The listing builds one solid part. Answer for the finished solid, in the listing's coordinates (mm). Face numbers are marked on the shaded views. A direction names the side the tool comes from. Coordinates: 2 decimals unless noted, no trailing zeros. Order: outer loops, then holes, each group sorted by start corner. A loop starts at its lowest first (then second) coordinate and runs counter-clockwise, first axis right, second up. Notation, with made-up numbers: (63.25, 71.5) -> (94.25, 71.5) arc R29 cw to (94.25, 110.5) -> close; hole circle Ø5 at (83, 7.5). An arc over 180 degrees is marked (long way). Return JSON: item names as keys, results as strings.
from build123d import *

# Parameters (mm, degrees)
SCHIZZO1_W                   = 20
SCHIZZO1_H                   = 15
SCHIZZO1_R                   = 1.75
ESTRUSIONE_ESTRUSIONE1_DEPTH = 5
SCHIZZO3_W                   = 20
SCHIZZO3_H                   = 5
ESTRUSIONE_ESTRUSIONE2_DEPTH = 13.5
SCHIZZO4_W                   = 20
SCHIZZO4_H                   = 5
ESTRUSIONE_ESTRUSIONE3_DEPTH = 17
RACCORDO1_R                  = 1


with BuildPart() as part:
    # Schizzo1 → Estrusione-Estrusione1 (new body)
    with BuildSketch(Plane.XY):
        Rectangle(SCHIZZO1_W, SCHIZZO1_H)
        with Locations((0, 2.5)):
            Circle(SCHIZZO1_R, mode=Mode.SUBTRACT)
    extrude(amount=ESTRUSIONE_ESTRUSIONE1_DEPTH)

    # Schizzo3 → Estrusione-Estrusione2 (add)
    with BuildSketch(Plane(origin=(0, 0, 0), x_dir=(-1, 0, 0), z_dir=(0, 0, -1))):
        with Locations((0, -5)):
            Rectangle(SCHIZZO3_W, SCHIZZO3_H)
    extrude(amount=ESTRUSIONE_ESTRUSIONE2_DEPTH)

    # Schizzo4 → Estrusione-Estrusione3 (add)
    with BuildSketch(Plane(origin=(0, -2.5, 0), x_dir=(1, 0, 0), z_dir=(0, 1, 0))):
        with Locations((0, 11)):
            Rectangle(SCHIZZO4_W, SCHIZZO4_H)
    extrude(amount=ESTRUSIONE_ESTRUSIONE3_DEPTH)

    # Raccordo1
    raccordo1_edges = [part.edges().sort_by_distance(p)[0] for p in [
        (0, -7.5, 5),
        (0, -7.5, -13.5),
        (0, 14.5, -13.5),
    ]]
    fillet(raccordo1_edges, radius=RACCORDO1_R)


solid = part.part
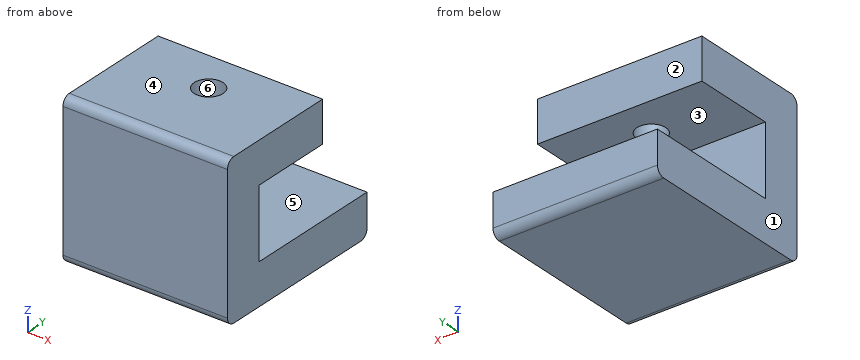
1. The part is cut by section A-A on y = 2.5. Give the vertices of the cut face in (x, z).
Answer block:
{"outline": "(-10, -13.5) -> (10, -13.5) -> (10, -8.5) -> (-10, -8.5) -> close; (-10, 0) -> (-1.75, 0) -> (-1.75, 5) -> (-10, 5) -> close; (1.75, 0) -> (10, 0) -> (10, 5) -> (1.75, 5) -> close"}
2. Determine the mould class of the marked faces 4, 5 and 6 for opening direction Z: pulls with the +Z half, pulls with the -Z half, needs draft (parallel to the pull), parting line crosses it, or undercut.
Answer block:
{"face 4": "pulls with the +Z half", "face 5": "undercut", "face 6": "needs draft"}
3. For the marked faces 1, 2 and 3, determine the directions among +Z, -Z, +X, -X, +Y, -Y from which every point of the face is accessible in a straight line to the end or side of a thin tool.
Answer block:
{"face 1": "+Z, -Z, -X, +Y, -Y", "face 2": "+Z, +X, -X, +Y", "face 3": "+X, -X, +Y"}
4. Each of these flat-tipped pins is pushed along its axis until it touches: pin 1 Ø4 at (y, z) = (10, 1.5) entering from +X; pin 2 Ø2.5 at (x, z) = (1.5, 3.5) entering from +Y; pin 3 Ø4 at (x, z) = (2, -6) entering from +Y. Where does it stop, or does it pass through?
Answer block:
{"pin 1": "passes through", "pin 2": "stops at y = 7.5", "pin 3": "stops at y = -2.5"}
5. The part is cut by section B-B on x = 0. Give the vertices of the cut face in (y, z), and give its area (3 significant figures).
Answer block:
{"outline": "(-7.5, -12.5) arc R1 ccw to (-6.5, -13.5) -> (13.5, -13.5) arc R1 ccw to (14.5, -12.5) -> (14.5, -8.5) -> (-2.5, -8.5) -> (-2.5, 0) -> (0.75, 0) -> (0.75, 5) -> (-6.5, 5) arc R1 ccw to (-7.5, 4) -> close; (4.25, 0) -> (7.5, 0) -> (7.5, 5) -> (4.25, 5) -> close", "area": "209 mm2"}
6. Consider line 1 (Y direction, x = 0, z = 2.55); line 2 (Z direction, x = 3.5, y = -1.75); line 3 (Y direction, x = -6.75, z = -5.25). Determine where each line is inside the solid, lowest interval first. Write a range as from..to.
Answer block:
{"line 1": "y = -7.5..0.75, 4.25..7.5", "line 2": "z = -13.5..-8.5, 0..5", "line 3": "y = -7.5..-2.5"}
7. The part is cut by section D-D on y = 5. Give the vertices of the cut face in (x, z), and give its area (3 significant figures).
Answer block:
{"outline": "(-10, -13.5) -> (10, -13.5) -> (10, -8.5) -> (-10, -8.5) -> close; (-10, 0) -> (10, 0) -> (10, 5) -> (-10, 5) -> close", "area": "200 mm2"}
8. The part is cut by section C-C on z = 2.25. Give the vertices of the cut face in (x, y).
Answer block:
{"outline": "(-10, -7.5) -> (10, -7.5) -> (10, 7.5) -> (-10, 7.5) -> close; hole circle Ø3.5 at (0, 2.5)"}
